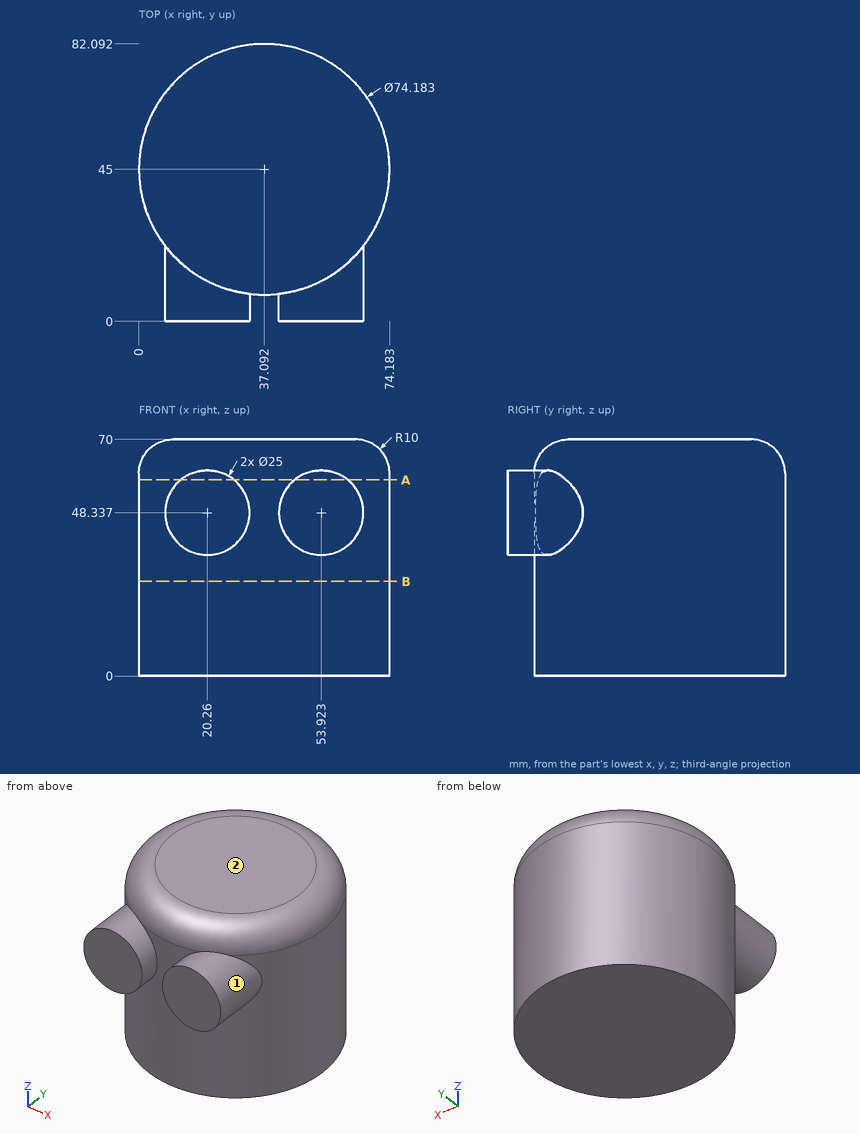
Study the drawing (mm; zero at the part's minimum x, y, z) and answer. A direction names the side the tool comes from. Round coordinates to 2 decimals unless told otherwise and drop trailing zeros. Loops run counter-clockwise (first coordinate to the right, second up) from the corner with the lowest first, then second, coordinate; pieces in that order, holes last. Notation, with made-up numbers: M 36,36 L 65,36 A20 ccw 65,57 Z; hole C -31.75,-22 d3. An arc over 180 degrees is marked long. One line per question, with ' | ' between items.
Q1. Each of these flat-tipped pins is pushed along its axis until it touches: pin 1 Ø5 at (x, z) = (11, 14.5) entering from +Y; pin 2 Ø4 at (x, y) = (63, 65.5) entering from +Z; pin 3 Ø8 at (x, z) = (50.5, 9.5) entering from -Y. Where does it stop, or does it pass through?
Conclusion:
pin 1: stops at y = 73.62 | pin 2: stops at z = 69.19 | pin 3: stops at y = 9.12
Q2. A tool of negligible diameter and unlimited length cuts with its end or side. For the marked faces 1 and 2, from which of +Z, -Z, +X, -X, +Y, -Y can it reach the whole face along a straight path? Write none if from no direction.
Conclusion:
face 1: -Y | face 2: +Z, +X, -X, +Y, -Y
Q3. Consider line 1 along X through (y, z) = (22, 49) (1 decimal); line 2 along Y through (x, z) = (30.5, 51.5); line 3 along Y through (x, z) = (17.5, 22) (1 decimal). Determine where each line is inside the solid, lowest interval first. Write a range as from..to.
Conclusion:
line 1: x = 7.8..66.4 | line 2: y = 0..81.5 | line 3: y = 13.5..76.5
Q4. Find section B-B, the plane z = 28. Give the vertices of the cut face in (x, y).
Conclusion:
outline: C 37.09,45 d74.18
Q5. Find section A-A, the plane z = 58. Give the vertices of the cut face in (x, y) (1 decimal).
Conclusion:
outline: M 12.3,0 L 28.2,0 L 28.2,9 A37.1 ccw 46,9 L 46,0 L 61.9,0 L 61.9,17.4 A37.1 ccw long 12.3,17.4 Z
